Source: CAD feature listing. Evaluate the final solid. Frame: model axes, mm. Give positions to 0.01 mm unless a question says otherwise; leave off trailing zeros. Order: outer loops, then holes, each group sorted by start corner. A loop starts at its lowest first (then second) coordinate and runs counter-clockwise, first axis right, second up. Notation, with made-up numbers: (81.5, 30.5) - (138.5, 30.5) arc R19 ccw to (138.5, 37.5) - close; hole circle Ø3 at (85.25, 13.25). An arc over 180 degrees is marked (long way). Use CSV: the item, a comma, the result in double quotes.
```python
from build123d import *

# Parameters (mm, degrees)
F0_W     = 605
F0_H     = 595
F1_DEPTH = 18
F2_SIZE  = 17.99999


# Not quite as in the source:
# - a fillet or chamfer is up to 0.001 mm smaller than in the source, because OpenCascade refuses the exact size


with BuildPart() as f1:
    # F0 (on Top) → F1 (new body)
    with BuildSketch(Plane.XY):
        with Locations((2.1061599255, 30.7130831559)):
            Rectangle(F0_W, F0_H)
    extrude(amount=-F1_DEPTH)

    # F2 (size 18 in the source; OpenCascade refuses exactly that, so slightly less here)
    f2_edges = [f1.edges().sort_by_distance(p)[0] for p in [
        (-300.39384, 30.713083, -18),
        (304.60616, 30.713083, -18),
    ]]
    chamfer(f2_edges, length=F2_SIZE)


solid = f1.part
```
Item 1: First-contact query: pin 1 (3 mm diameter, centred on y = 117.5, z = -13, fed in from -X). Flat tip, straight axial feed; report the tip coordinate or a pass-through.
Filled in:
pin 1,"stops at x = -288.89"
Item 2: Mould query, pull axis Z, two halves, no side actions, for faces 1 (the flat face through (295.48, 26.548, -9.126)), 2 (the flat face through (-2, 35, 0)), 3 (the flat face through (-2, 328.213, -9)). Classes: released by +Z, released by -Z, zero draft, split by the parting line, or undercut.
Filled in:
face 1,"released by -Z"
face 2,"released by +Z"
face 3,"zero draft"
Item 3: Section B-B on z = -10. Return the cut outline in (x, y).
Filled in:
outline,"(-290.39, -266.79) - (294.61, -266.79) - (294.61, 328.21) - (-290.39, 328.21) - close"
Item 4: Material intervals for line 1 (X direction, y = 10.5, z = -1); line 2 (X direction, y = 250.5, z = -10), sorted ascending. Write a range as from..to.
Filled in:
line 1,"x = -299.39..303.61"
line 2,"x = -290.39..294.61"
